Answer from the drawing. Dimensions are ordinates in mm from the lowest x, y and z of the part. A direction names the side the tool comes from. Round coordinates to 2 decimals unless told otherwise and drop trailing zeros. Write each loop counter-clockwise with the first axis right and the second up, starting at its lowest first coordinate (ties: lowest second). Pieces come first, ordered by that corner, then holes. Notation, with made-up numbers: (-34, -4.5) - (5, -4.5) arc R13 ccw to (5, 2.5) - close; hole circle Ø5 at (89.25, -2.75). An arc over 180 degrees is marked (long way). Answer in a Markdown table with one row per item.
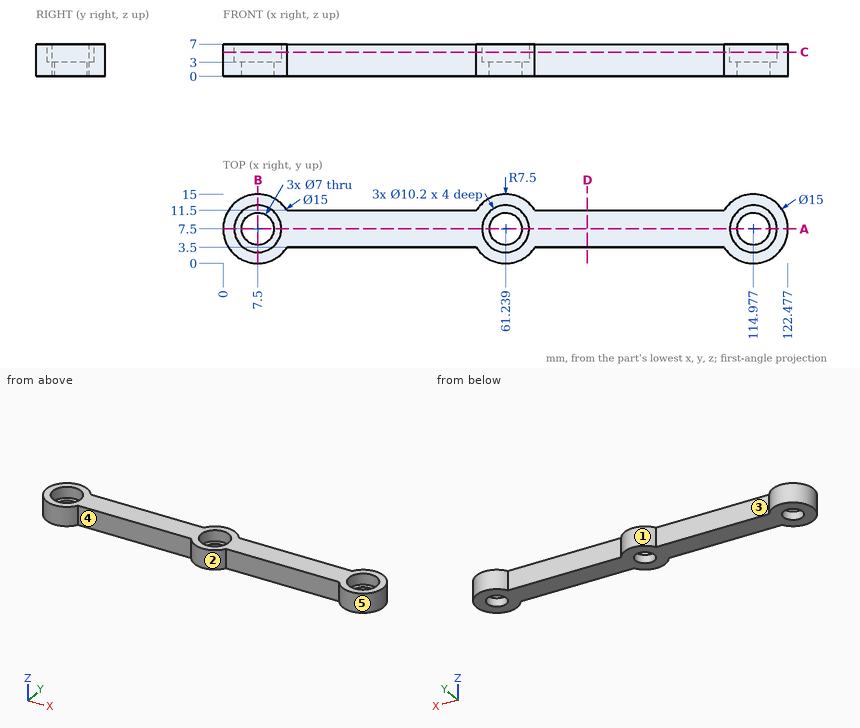
(1) Find the intervals of material crossed by line 1 (X direction, y = 7.25, z = 6.75) (1 decimal); line 2 (X direction, y = 13, z = 4) (1 decimal); line 3 (Y direction, x = 7.5, z = 4.55), in increasing order.
Checked values:
| item | result |
|---|---|
| line 1 | x = 0 to 2.4, 12.6 to 56.1, 66.3 to 109.9, 120.1 to 122.5 |
| line 2 | x = 2.4 to 12.6, 56.1 to 66.3, 109.9 to 120.1 |
| line 3 | y = 0 to 2.4, 12.6 to 15 |
(2) Section A-A (y = 7.5) is taken. Give the vertices of the cut face in (x, z).
Checked values:
| item | result |
|---|---|
| outline | (0, 0) - (4, 0) - (4, 3) - (2.4, 3) - (2.4, 7) - (0, 7) - close; (11, 0) - (57.74, 0) - (57.74, 3) - (56.14, 3) - (56.14, 7) - (12.6, 7) - (12.6, 3) - (11, 3) - close; (64.74, 0) - (111.48, 0) - (111.48, 3) - (109.88, 3) - (109.88, 7) - (66.34, 7) - (66.34, 3) - (64.74, 3) - close; (118.48, 0) - (122.48, 0) - (122.48, 7) - (120.08, 7) - (120.08, 3) - (118.48, 3) - close |
(3) Flat-ended cylindrical pins translate along their axes: pin 1 (8 mm diameter, centred on x = 61.24, y = 7.5, fed in from +Z); pin 2 (1 mm diameter, centred on x = 56, z = 4, fed in from -Y); pin 3 (2 mm diameter, centred on x = 83.5, z = 1.5, fed in from -Y). Find the tip coordinate at first contact, or state that the pin passes through.
Checked values:
| item | result |
|---|---|
| pin 1 | stops at z = 3 |
| pin 2 | stops at y = 1.69 |
| pin 3 | stops at y = 3.5 |
(4) For the marked faces 3, 4 and 5, determine the directions among +Z, -Z, +X, -X, +Y, -Y from which every point of the face is accessible in a straight line to the end or side of a thin tool.
Checked values:
| item | result |
|---|---|
| face 3 | +Z, -Z, +Y |
| face 4 | +Z, -Z, -Y |
| face 5 | +Z, -Z |
(5) Section C-C (z = 5.25) is taken. Give the vertices of the cut face in (x, y) (1 decimal).
Checked values:
| item | result |
|---|---|
| outline | (13.8, 3.5) - (54.9, 3.5) arc R7.5 ccw to (67.6, 3.5) - (108.6, 3.5) arc R7.5 ccw (long way) to (108.6, 11.5) - (67.6, 11.5) arc R7.5 ccw to (54.9, 11.5) - (13.8, 11.5) arc R7.5 ccw (long way) to start; hole circle Ø10.2 at (7.5, 7.5); hole circle Ø10.2 at (61.2, 7.5); hole circle Ø10.2 at (115, 7.5) |
(6) Section D-D (x = 79) is taken. Give the vertices of the cut face in (y, z), and give its area (3 significant figures).
Checked values:
| item | result |
|---|---|
| outline | (3.5, 0) - (11.5, 0) - (11.5, 7) - (3.5, 7) - close |
| area | 56.0 mm2 |
(7) Section B-B (x = 7.5) is taken. Give the vertices of the cut face in (y, z).
Checked values:
| item | result |
|---|---|
| outline | (0, 0) - (4, 0) - (4, 3) - (2.4, 3) - (2.4, 7) - (0, 7) - close; (11, 0) - (15, 0) - (15, 7) - (12.6, 7) - (12.6, 3) - (11, 3) - close |
(8) For a pull along X with two mould halves and no side action, classify the marked faces 1 and 2 as pulls with the +X half, pulls with the -X half, needs draft (parallel to the pull), parting line crosses it, or undercut.
Checked values:
| item | result |
|---|---|
| face 1 | undercut |
| face 2 | undercut |
